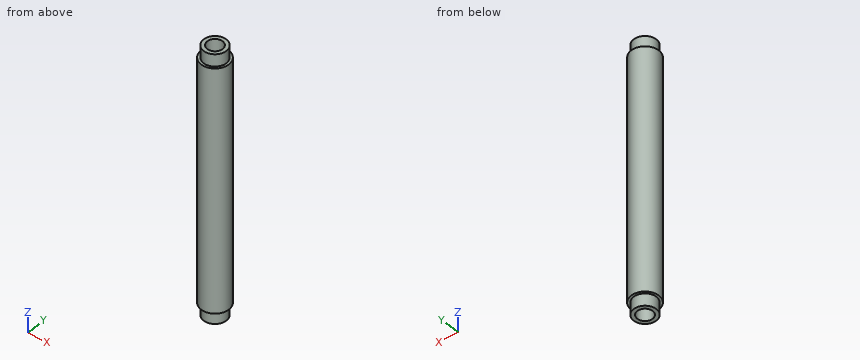
```python
from build123d import *

# Parameters (mm, degrees)
F0_R     = 5.715
F0_R_2   = 3.175
F1_DEPTH = 100
F2_R     = 4.70576
F2_R_2   = 3.175
F3_DEPTH = 5
F4_R     = 4.70576
F4_R_2   = 3.175
F5_DEPTH = 5


with BuildPart() as f1:
    # F0 (on Top) → F1 (new body)
    with BuildSketch(Plane.XY):
        Circle(F0_R)
        Circle(F0_R_2, mode=Mode.SUBTRACT)
    extrude(amount=F1_DEPTH)

    # F2 (on face) → F3 (join)
    with BuildSketch(Plane.XY.offset(100)):
        Circle(F2_R)
        Circle(F2_R_2, mode=Mode.SUBTRACT)
    extrude(amount=F3_DEPTH)

    # F4 (on Top) → F5 (join)
    with BuildSketch(Plane.XY):
        Circle(F4_R)
        Circle(F4_R_2, mode=Mode.SUBTRACT)
    extrude(amount=-F5_DEPTH)


solid = f1.part
```
Could you check a few things on this model? Use its own coordinates, in mm. Round coordinates to 2 decimals unless told otherwise and drop trailing zeros. Write each loop counter-clockwise with the first axis right and the second up, starting at its lowest first coordinate (ties: lowest second). Pieces come first, ordered by that corner, then holes.
(1) Suppose I cut it at C-C on z = 81. Write out the boundary of the cut face in (x, y) (3 decimals).
Findings below:
outline: circle Ø11.43 at (0, 0); hole circle Ø6.35 at (0, 0)
(2) If I drill on probe 1 along Y at (x, z) = (0, 24.5) (3 decimals); probe 2 along X at (y, z) = (1.5, 70); probe 3 along X at (y, z) = (2.25, 74), over which ranges is the centre line in solid material (lowest first)?
Findings below:
probe 1: y = -5.715 to -3.175, 3.175 to 5.715
probe 2: x = -5.51 to -2.8, 2.8 to 5.51
probe 3: x = -5.25 to -2.24, 2.24 to 5.25
(3) Suppose I cut it at A-A on y = 0. Write out the boundary of the cut face in (x, z) (3 decimals), and give its area (3 significant figures).
Findings below:
outline: (-5.715, 0) - (-4.706, 0) - (-4.706, -5) - (-3.175, -5) - (-3.175, 105) - (-4.706, 105) - (-4.706, 100) - (-5.715, 100) - close; (3.175, -5) - (4.706, -5) - (4.706, 0) - (5.715, 0) - (5.715, 100) - (4.706, 100) - (4.706, 105) - (3.175, 105) - close
area: 539 mm2
(4) For pin 1 (1 mm diameter, centred on x = 4, y = 4.5, fed in from +Z); pin 2 (2 mm diameter, centred on x = 1.5, z = 29, fed in from -Y); pin 3 (5 mm diameter, centred on y = 3, z = 27, fed in from +X), each with a flat end and sliding along its axis, tell me the tip position at first contact or that it passes through.
Findings below:
pin 1: stops at z = 100
pin 2: stops at y = -5.69
pin 3: stops at x = 5.69
